from build123d import *

# Parameters (mm, degrees)
BOSS_EXTRUDE1_DEPTH      = 6
BOSS_EXTRUDE1_DEPTH_BACK = 33
SKETCH1_R                = 18
SKETCH1_R_2              = 6.35
CUT_EXTRUDE1_OUTLINE_W   = 2
CUT_EXTRUDE1_OUTLINE_H   = 11.973288181
CIRPATTERN1_COUNT        = 2
SKETCH2_OUTSIDE_W        = 50.826
SKETCH2_OUTSIDE_H        = 50.826
SKETCH2_OUTSIDE_R        = 12.15
CUT_EXTRUDE2_DEPTH       = 34


# Read off the part's stored shape, not the designer's step: Cut-Extrude1
with BuildPart() as part:
    # Sketch1 → Boss-Extrude1 (new, two sides: drawn at the far end of the back side and taken through both)
    with BuildSketch(Plane.XY.offset(-BOSS_EXTRUDE1_DEPTH_BACK)):
        Circle(SKETCH1_R)
        Circle(SKETCH1_R_2, mode=Mode.SUBTRACT)
    extrude(amount=BOSS_EXTRUDE1_DEPTH + BOSS_EXTRUDE1_DEPTH_BACK)

    # Cut-Extrude1 outline → Cut-Extrude1 (revolve, cut)
    with BuildSketch(Plane.YX.offset(-3.5)):
        with Locations((1, -12.013415915)):
            Rectangle(CUT_EXTRUDE1_OUTLINE_W, CUT_EXTRUDE1_OUTLINE_H)
    cut_extrude1 = revolve(axis=Axis((0, 0, 3.5), (1, 0, 0)), mode=Mode.SUBTRACT)

    # CirPattern1: Cut-Extrude1 ×2 about axis
    cirpattern1_axis = Axis((0, 0, 6), (0, 0, 1))
    for i in range(1, CIRPATTERN1_COUNT):
        add(cut_extrude1.rotate(cirpattern1_axis, i * 360 / CIRPATTERN1_COUNT), mode=Mode.SUBTRACT)

    # Sketch2 outside → Cut-Extrude2 (cut)
    with BuildSketch(Plane(origin=(0, 0, -33), x_dir=(-1, 0, 0), z_dir=(0, 0, -1))):
        Rectangle(SKETCH2_OUTSIDE_W, SKETCH2_OUTSIDE_H)
        Circle(SKETCH2_OUTSIDE_R, mode=Mode.SUBTRACT)
    extrude(amount=-CUT_EXTRUDE2_DEPTH, mode=Mode.SUBTRACT)


solid = part.part
Check sheet for the modelled part. Datum: model origin and axes. Units: mm. A direction names the side the tool comes from. Round coordinates to 2 decimals unless told otherwise and drop trailing zeros. Order: outer loops, then holes, each group sorted by start corner. A loop starts at its lowest first (then second) coordinate and runs counter-clockwise, first axis right, second up.
(1) Cross-section at A-A, the plane x = 0. Enter the section's corners in (y, z).
(2) Cross-section at C-C, the plane z = -5. Enter the section's corners in (x, y).
(3) Draft check along X on faces 1 (the cylindrical face through (-1.38, -6.2, -13.77)), 2 (the cylindrical face through (11.93, -1.908, 4.101)), 3 (the cylindrical face through (17.169, 5.407, 3.465)). Enter one of: pulls with the +X half, pulls with the -X half, needs draft (parallel to the pull), parting line crosses it, or undercut.
(4) Access from +Z, -Z, +X, -X, +Y, -Y to the whole of each face (thin tool, end or side, straight path). Record for faces 4 (the flat face through (0, -8, 6)), 5 (the flat face through (-4, -12, 1)).
(5) Scan lines: probe 1 along Y at (x, z) = (0, -4); probe 2 along X at (y, z) = (-2, -20.5); probe 3 along X at (y, z) = (-2.5, 1.5). Record each from-to range of solid material in increasing order.
(6) Cross-section at D-D, the plane x = 11.5. Enter the section's corners in (y, z), and give its area (3 significant figures).
(7) Go/stop test with flat-tipped pins: P1, Ø4, axis at x = -2, z = -7, coming from the -Y side; P2, Ø1, axis at y = -4, z = -11, coming from the +X side; P3, Ø8, axis at x = 9.5, z = -1, coming from the +Y side. Record where each tip stops, or that it passes through.
(8) Cross-section at B-B, the plane y = 0. Enter the section's corners in (x, z).
Check sheet entries:
1. outline: (-18, 1) - (-12.15, 1) - (-12.15, -33) - (-6.35, -33) - (-6.35, 6) - (-18, 6) - close; (6.35, -33) - (12.15, -33) - (12.15, 1) - (18, 1) - (18, 6) - (6.35, 6) - close
2. outline: circle Ø24.3 at (0, 0); hole circle Ø12.7 at (0, 0)
3. face 1: undercut
3. face 2: needs draft
3. face 3: parting line crosses it
4. face 4: +Z, +X, -X, +Y, -Y
4. face 5: -Z
5. probe 1: y = -12.15 to -6.35, 6.35 to 12.15
5. probe 2: x = -11.98 to -6.03, 6.03 to 11.98
5. probe 3: x = -17.83 to -5.84, 5.84 to 17.83
6. outline: (-13.85, 1) - (-3.92, 1) - (-3.92, -33) - (3.92, -33) - (3.92, 1) - (13.85, 1) - (13.85, 6) - (-13.85, 6) - close; hole circle Ø4 at (0, 3.5)
6. area: 393 mm2
7. P1: stops at y = -12.15
7. P2: stops at x = 11.63
7. P3: stops at y = 16.96
8. outline: (-18, 1) - (-12.15, 1) - (-12.15, -33) - (-6.35, -33) - (-6.35, 1.5) - (-18, 1.5) - close; (-18, 5.5) - (-6.35, 5.5) - (-6.35, 6) - (-18, 6) - close; (6.35, -33) - (12.15, -33) - (12.15, 1) - (18, 1) - (18, 1.5) - (6.35, 1.5) - close; (6.35, 5.5) - (18, 5.5) - (18, 6) - (6.35, 6) - close
